Part print with two shaded views. Sizes in mm from the minimum x, y, z corner. Coordinates: 2 decimals unless noted, no trailing zeros. Write each loop counter-clockwise with the first axis right and the second up, starting at its lowest first coordinate (ties: lowest second). Pieces come first, ordered by that corner, then holes.
Q1. Band-saw the part on D-D, the plane x = 7. Write the cut outline in (y, z), plus the area to 3 significant figures.
Q2. Band-saw the part on A-A, the plane y = 3. Write the cut outline in (x, z), plus the area to 3 significant figures.
Q3. Drill centre lines: probe 1 along Z at (x, y) = (65.9, 3.85); probe 2 along X at (y, z) = (5.75, 51.25); probe 3 along X at (y, z) = (4.1, 18.65). Where is each one in solid material? Low to high.
Q4. Band-saw the part on B-B, the plane x = 65.9. Write the cut outline in (y, z), plus the area to 3 significant figures.
Q5. Band-saw the part on C-C, the plane z = 46.55. Write the cut outline in (x, y).
Q6. Pin check, flat tip, straight feed: P1, Ø6, axis at x = 12.5, z = 23, coming from the +Y side. Stop position of the tip, or through.
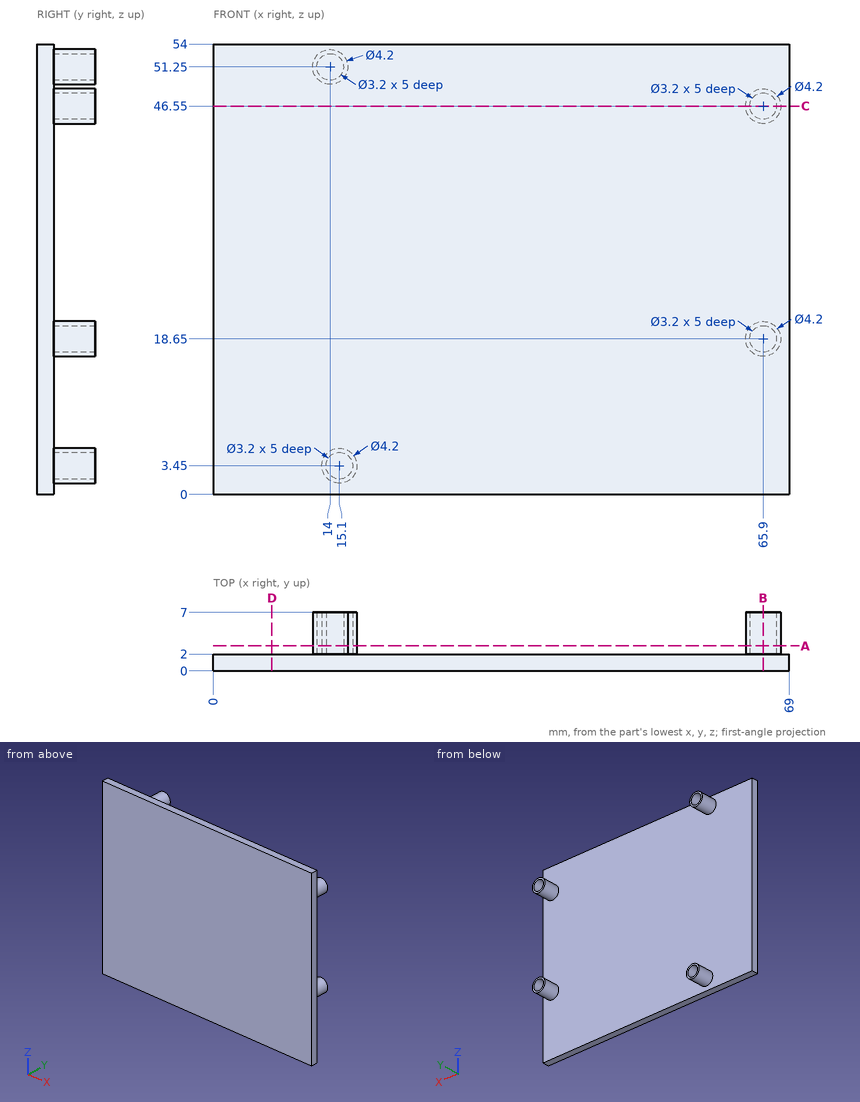
Answer sheet:
1. outline: (0, 0) - (2, 0) - (2, 54) - (0, 54) - close
1. area: 108 mm2
2. outline: circle Ø4.2 at (14, 51.25); circle Ø4.2 at (15.1, 3.45); circle Ø4.2 at (65.9, 18.65); circle Ø4.2 at (65.9, 46.55); hole circle Ø3.2 at (14, 51.25); hole circle Ø3.2 at (15.1, 3.45); hole circle Ø3.2 at (65.9, 18.65); hole circle Ø3.2 at (65.9, 46.55)
2. area: 23.2 mm2
3. probe 1: z = 16.55 to 17.05, 20.25 to 20.75, 44.45 to 44.95, 48.15 to 48.65
3. probe 2: x = 11.9 to 12.4, 15.6 to 16.1
3. probe 3: x = 63.8 to 64.3, 67.5 to 68
4. outline: (0, 0) - (2, 0) - (2, 16.55) - (7, 16.55) - (7, 17.05) - (2, 17.05) - (2, 20.25) - (7, 20.25) - (7, 20.75) - (2, 20.75) - (2, 44.45) - (7, 44.45) - (7, 44.95) - (2, 44.95) - (2, 48.15) - (7, 48.15) - (7, 48.65) - (2, 48.65) - (2, 54) - (0, 54) - close
4. area: 118 mm2
5. outline: (0, 0) - (69, 0) - (69, 2) - (68, 2) - (68, 7) - (67.5, 7) - (67.5, 2) - (64.3, 2) - (64.3, 7) - (63.8, 7) - (63.8, 2) - (0, 2) - close
6. P1: stops at y = 2
